Here's how the part is built. I have some questions about the finished solid (model axes, mm). A direction names the side the tool comes from. Coordinates: 2 decimals unless noted, no trailing zeros. Write each loop counter-clockwise with the first axis right and the second up, starting at its lowest first coordinate (ties: lowest second). Pieces come first, ordered by that corner, then holes. Notation, with made-up numbers: (-21.5, -26.5) -> (-11.5, -26.5) arc R26 cw to (-11.5, -9.5) -> close; hole circle Ø8 at (52, -19.75). An arc over 180 degrees is marked (long way). Put each result on its own line as item: value. Start each with the question number.
Item 1: For pin 1 (8 mm diameter, centred on x = -15, y = -29.5, fed in from -Z); pin 2 (4 mm diameter, centred on y = 16.5, z = 12, fed in from -X); pin 3 (2 mm diameter, centred on x = 20, z = 31, fed in from -Y), each with a flat end and sliding along its axis, tell me the tip position at first contact or that it passes through.
Item 2: On a 3-axis mill with a long thin cutter (end or side, diameter ignored), from which of +Z, -Z, +X, -X, +Y, -Y can I reach the whole of each face in a straight line? I mean faces 4 (the face through (-35.96, 35.8, -37.53)), 5 (the face through (-37, 0, -38)). Say none if no direction works.
Item 3: I want a section at C-C, the plane y = -21.5. List the corners of the cut face in (x, z) for me, then the cut area to 3 significant figures.
Item 4: I want a section at D-D, the plane z = 28. List the corners of the cut face in (x, y) for me.
Item 5: I want a section at A-A, the plane x = 13. List the corners of the cut face in (y, z) for me, then the cut area to 3 significant figures.
Item 6: I want a section at B-B, the plane z = -10.5. List the corners of the cut face in (x, y) for me, then the cut area to 3 significant figures.
Item 7: If we mould it in two halves opening along Y, with no side actions, what happens to faces 1 (the face through (-39, 0, -39)), 2 (the face through (33.8, 33.96, -2.6)), 3 (the face through (35.96, -35.8, -19.01))? For each: released by +Y, released by -Y, zero draft, split by the parting line, or undercut.
Item 8: I need wall thicknesses on line 1 (Y direction, x = 11.5, z = -14); line 2 (X direction, y = 23, z = -5). Which ranges of each line are inside material? Lowest first, please. Write a range as [from, to].
from build123d import *

# Parameters (mm, degrees)
SKETCH1_W           = 78
SKETCH1_H           = 78
SKETCH1_W_2         = 74
SKETCH1_H_2         = 74
BOSS_EXTRUDE1_DEPTH = 50
FILLET1_R           = 10.65
CUT_EXTRUDE1_DEPTH  = 101.523629063
CUT_EXTRUDE2_DEPTH  = 101.523629063


with BuildPart() as part:
    # Sketch1 → Boss-Extrude1 (new, symmetric)
    with BuildSketch(Plane.XY):
        Rectangle(SKETCH1_W, SKETCH1_H)
        Rectangle(SKETCH1_W_2, SKETCH1_H_2, mode=Mode.SUBTRACT)
    extrude(amount=BOSS_EXTRUDE1_DEPTH, both=True)

    # Fillet1
    fillet1_edges = [part.edges().sort_by_distance(p)[0] for p in [
        (37, -37, 0),
        (37, 37, 0),
        (-37, 37, 0),
        (-37, -37, 0),
        (39, -39, 0),
        (-39, -39, 0),
        (-39, 39, 0),
        (39, 39, 0),
    ]]
    fillet(fillet1_edges, radius=FILLET1_R)

    # Sketch2 → Cut-Extrude1 (cut, through all)
    with BuildSketch(Plane(origin=(39, 0, 0), x_dir=(0, 0, -1), z_dir=(1, 0, 0))):
        Polygon((-50, 39), (-50, -39), (-4.966679003, -39), align=None)
    extrude(amount=-CUT_EXTRUDE1_DEPTH, mode=Mode.SUBTRACT)

    # Sketch3 → Cut-Extrude2 (cut, through all)
    with BuildSketch(Plane(origin=(0, 39, 0), x_dir=(1, 0, 0), z_dir=(0, 1, 0))):
        Polygon((-39, -50), (39, -50), (-39, 28), align=None)
    extrude(amount=-CUT_EXTRUDE2_DEPTH, mode=Mode.SUBTRACT)


solid = part.part
Calculated:
1. pin 1: passes through
1. pin 2: stops at x = 37
1. pin 3: stops at y = 37
2. face 4: +Z, -Z, -X, +Y
2. face 5: +Z, -Z
3. outline: (-39, -50) -> (-37, -50) -> (-37, -26) -> (-39, -28) -> close; (37, -50) -> (39, -50) -> (39, 15.07) -> (37, 15.07) -> close
3. area: 176 mm2
4. outline: (17, 37) -> (26.35, 37) arc R10.65 cw to (37, 26.35) -> (37, 0.89) -> (39, 0.89) -> (39, 28.35) arc R10.65 ccw to (28.35, 39) -> (17, 39) -> close
5. outline: (-39, -50) -> (-37, -50) -> (-37, 6.12) -> (-39, 4.97) -> close; (37, -50) -> (39, -50) -> (39, 24) -> (37, 24) -> close
5. area: 259 mm2
6. outline: (-21.5, -39) -> (28.35, -39) arc R10.65 ccw to (39, -28.35) -> (39, 28.35) arc R10.65 ccw to (28.35, 39) -> (-21.5, 39) -> (-21.5, 37) -> (26.35, 37) arc R10.65 cw to (37, 26.35) -> (37, -26.35) arc R10.65 cw to (26.35, -37) -> (-21.5, -37) -> close
6. area: 390 mm2
7. face 1: zero draft
7. face 2: undercut
7. face 3: released by -Y
8. line 1: y = [-39, -37], [37, 39]
8. line 2: x = [37, 39]
